Here's how the part is built. I have some questions about the finished solid (model axes, mm). A direction names the side the tool comes from. Give positions to 0.01 mm unless a question says otherwise; leave off trailing zeros. Loops run counter-clockwise (first coordinate to the right, second up) from the corner with the lowest first, then second, coordinate; pieces in that order, holes last. Notation, with made-up numbers: (-23.5, 30) -> (-1.5, 30) arc R31 ccw to (-1.5, 55) -> close; hole circle Ø5 at (28, -39). An arc over 180 degrees is marked (long way). Answer in a Markdown table with one row per item. Add a question column.
Item 1: If we section it at D-D (z = -50.5): Write out the boundary of the cut face in (x, y).
Item 2: Which directions (+Z, -Z, +X, -X, +Y, -Y) give clear straight access to the entire face, cutting with the end or side of a thin tool? Please do faces 4 (the face through (21, -23, 42.867)), 5 (the face through (7.4, -33.326, 50.916)), 6 (the face through (7.7, -30.2, 58.742)).
Item 3: For P1, Ø1.5, axis at y = -0.5, z = -4.5, coming from the +X side; P2, Ø10, axis at x = 18.5, z = 27.5, coming from the -Y side; P3, Ø2, axis at y = -11.5, z = -29, coming from the +X side, each with a flat end and sliding along its axis, tell me the tip position at first contact or that it passes through.
Item 4: We'd pull the mould along X, two halves only. Please class faces 1 (the face through (27.61, -21.17, -21.52)), 2 (the face through (0, 0, -84.133)), 3 (the face through (30.933, 1.361, 50.916)): released by +X, released by -X, zero draft, split by the parting line, or undercut.
Item 5: If we section it at C-C (z = -4.5): Write out the boundary of the cut face in (x, y), then the cut area to 3 significant figures.
Item 6: If I drill on line 1 (Y direction, x = 0, z = 46.5); line 2 (Z direction, x = 1.5, y = -12); line 3 (Y direction, x = -4.5, z = 4), over which ranges is the centre line in solid material (lowest first)?
Item 7: If we section it at A-A (y = 0): Write out the boundary of the cut face in (x, z).
```python
from build123d import *

# Parameters (mm, degrees)
F0_W = 3.175
F0_H = 15.875
F2_T = 2.54


# Not quite as in the source:
# - a shell that OpenCascade refuses in one call is made with other operations: the cavity is built on its own and cut out


with BuildPart() as f1:
    # F0 (on Front) → F1 (revolve)
    with BuildSketch(Plane.XZ):
        Polygon((0, -84.1329338265), (0, 42.8670661735), (-30.9626, 42.8670661735), (-34.1376, 42.8670661735), (-44.45, 42.8670661735), (-25.4, -84.1329338265), align=None)
        with Locations((-32.5501, 50.8045661735)):
            Rectangle(F0_W, F0_H)
    revolve(axis=Axis((0, 0, -17.2506261634), (0, 0, -1)))

    # F2: shell of thickness 2.54, made by hand


with BuildPart() as f2_core1:
    # F2_t2: copy of F1
    add(f1.part)

    # the walls: a layer under each face that stays
    f2_faces = [f2_core1.faces().sort_by_distance(p)[0] for p in [
        (30.9626, 0, 50.8045661735),
        (-22.7584, -22.7584, 58.7420661735),
        (34.1376, 0, 50.8045661735),
        (-29.6333333333, -29.6333333333, 42.8670661735),
        (34.925, 0, -20.6329338265),
        (0, 0, -84.1329338265),
    ]]
    thicken(f2_faces, amount=-F2_T, mode=Mode.SUBTRACT)

    # F2_s3 → F2_t4 (revolve, cut)
    with BuildSketch(Plane.XZ):
        Polygon((-34.163, 42.8924661735), (-31.5976, 42.8670661735), (-31.5976, 40.3270661735), (-34.1376, 40.3270661735), align=None)
    revolve(axis=Axis((0, 0, 42.8670661735), (0, 0, -1)), mode=Mode.SUBTRACT)


with BuildPart() as f1_1:
    add(f1.part)

    # what is left inside the walls is the cavity
    f2_cavity = [f2_core1.part.solids().sort_by_distance(p)[0] for p in [
        (35.379465, 0, -0.309166),
    ]]
    add(f2_cavity, mode=Mode.SUBTRACT)


solid = f1_1.part
```
Recorded:
| question | item | result |
|---|---|---|
| 1 | outline | circle Ø60.89 at (0, 0); hole circle Ø55.75 at (0, 0) |
| 2 | face 4 | none |
| 2 | face 5 | +Z |
| 2 | face 6 | +Z, +X, -X, +Y, -Y |
| 3 | P1 | stops at x = 37.45 |
| 3 | P2 | stops at y = -40.1 |
| 3 | P3 | stops at x = 32.03 |
| 4 | face 1 | split by the parting line |
| 4 | face 2 | zero draft |
| 4 | face 3 | undercut |
| 5 | outline | circle Ø74.69 at (0, 0); hole circle Ø69.55 at (0, 0) |
| 5 | area | 582 mm^2 |
| 6 | line 1 | y = -34.14 to -30.96, 30.96 to 34.14 |
| 6 | line 2 | z = -84.13 to -81.59 |
| 6 | line 3 | y = -38.36 to -35.77, 35.77 to 38.36 |
| 7 | outline | (-44.45, 42.87) -> (-25.4, -84.13) -> (25.4, -84.13) -> (44.45, 42.87) -> (34.14, 42.87) -> (34.14, 58.74) -> (30.96, 58.74) -> (30.96, 42.87) -> (31.6, 42.87) -> (31.6, 40.33) -> (41.5, 40.33) -> (23.21, -81.59) -> (-23.21, -81.59) -> (-41.5, 40.33) -> (-31.6, 40.33) -> (-31.6, 42.87) -> (-30.96, 42.87) -> (-30.96, 58.74) -> (-34.14, 58.74) -> (-34.14, 42.87) -> close |
